The figure shows three views and two pictorial views of one solid part (mm, origin at its lowest corner). Answer the questions. A direction names the side the tool comes from. Give positions to 0.01 mm unless a question says otherwise; leave off trailing zeros. Order: outer loops, then holes, each group sorted by start corner. A loop starts at its lowest first (then second) coordinate and runs counter-clockwise, first axis right, second up. Notation, with made-up numbers: (7.25, 25) -> (13.25, 25) arc R23 cw to (13.25, 44) -> close; hole circle Ø7 at (12.25, 67.5). An arc over 180 degrees is marked (long way). Use one line per item in the form item = value.
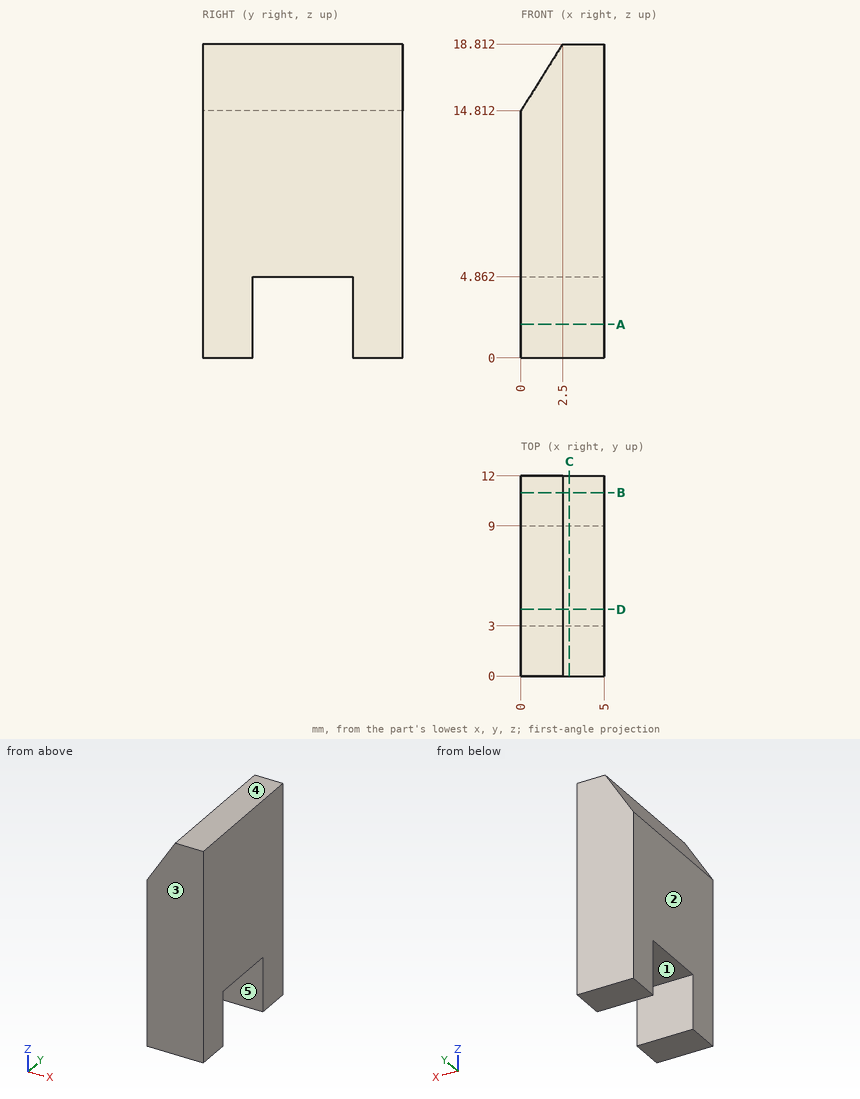
Item 1: Determine the mould class of the marked faces 1, 2 and 3 for opening direction Y: +Y half, -Y half, draft (parallel to the pull), parting line (faces both ways), or undercut.
Checks:
face_1 = undercut
face_2 = draft
face_3 = -Y half
Item 2: Straight lines are drawn through the part: L1, parallel to Y at x = 2.75, z = 2.25; L2, parallel to Z at x = 3.95, y = 8; L3, parallel to Z at x = 2.3, y = 8.5 (1 decimal). For each, find the intervals that lie inside material, in ascending order. Write a range as from..to.
Checks:
L1 = 0..3, 9..12
L2 = 4.86..18.81
L3 = 4.9..18.5
Item 3: The part is cut by section C-C on x = 2.9. Give the vertices of the cut face in (y, z), and give its area (3 significant figures).
Checks:
outline = (0, 0) -> (3, 0) -> (3, 4.86) -> (9, 4.86) -> (9, 0) -> (12, 0) -> (12, 18.81) -> (0, 18.81) -> close
area = 197 mm²
Item 4: Which of the six approach directions +Z, -Z, +X, -X, +Y, -Y give full straight-line access (tool end or side, diameter ignored) to the marked faces 4 and 5?
Checks:
face_4 = +Z, +X, -X, +Y, -Y
face_5 = -Z, +X, -X
Item 5: The part is cut by section A-A on z = 2. Give the vertices of the cut face in (x, y).
Checks:
outline = (0, 0) -> (5, 0) -> (5, 3) -> (0, 3) -> close; (0, 9) -> (5, 9) -> (5, 12) -> (0, 12) -> close
Item 6: The part is cut by section D-D on y = 4. Give the vertices of the cut face in (x, z).
Checks:
outline = (0, 4.86) -> (5, 4.86) -> (5, 18.81) -> (2.5, 18.81) -> (0, 14.81) -> close
Item 7: Given pin 1 Ø2.5 at (x, y) = (2.5, 5) entering from -Z, flat-ended and moving along its own axis, determine where the tip first touches the part or whether it passes through.
Checks:
pin_1 = 4.86
Item 8: The part is cut by section B-B on y = 11. Give the vertices of the cut face in (x, z).
Checks:
outline = (0, 0) -> (5, 0) -> (5, 18.81) -> (2.5, 18.81) -> (0, 14.81) -> close
